For this review, take the finished solid that the model builds, in its own axes (mm). A direction names the side the tool comes from. Round coordinates to 2 decimals unless told otherwise and drop trailing zeros. Write each loop counter-clockwise with the first axis right and the second up, starting at its lowest first coordinate (ties: lowest second). Pieces come first, ordered by that corner, then holes.
from build123d import *

# Parameters (mm, degrees)
F0_W     = 42.5292160362
F0_H     = 54.7678396106
F1_DEPTH = 25.4
F5_DEPTH = 12.7
F6_DEPTH = 12.7


with BuildPart() as f1:
    # F0 (on Right) → F1 (new body)
    with BuildSketch(Plane.YZ):
        with Locations((0.3059664741, 8.7200179696)):
            Rectangle(F0_W, F0_H)
    extrude(amount=F1_DEPTH)


with BuildPart() as f5:
    # F4 (on Front) → F5 (new body, symmetric)
    with BuildSketch(Plane.XZ):
        Polygon((7.8021222726, 46.5067662299), (-7.8021222726, 46.5067662299), (-15.1452962309, 44.0590418875), (-23.1004003435, 35.4920066893), (-25.8540920913, 30.2905943245), (-27.6898853481, 19.5817966014), (-27.3839198053, 5.8133457787), (-30.1376096904, 8.8730016723), (-32.5853340328, 7.9551050439), (-34.4211272895, 4.5894836076), (-34.1151617467, -1.8357934896), (-33.1972651184, -7.3431739584), (-30.4435752332, -11.6266915575), (-27.0779542625, -12.85055466), (-26.1600576341, -18.6639018357), (-23.7123332918, -24.7832108289), (-17.2870550305, -33.3502478898), (-10.8617777005, -43.1411489844), (-5.9663290158, -45.8948388696), (0.1529839792, -47.1187010407), (5.6603644043, -45.5888696015), (11.4582879852, -42.2321807174), (17.2870550305, -33.3502478898), (22.4884822373, -26.4150121165), (24.2018731435, -23.5593615721), (26.1600576341, -18.6639018357), (26.5130960305, -16.4279912753), (26.4660250396, -15.9102100879), (26.6190057487, -15.7572295118), (27.0779542625, -12.85055466), (30.4435752332, -11.6266915575), (33.1972651184, -7.3431739584), (34.1151617467, -1.8357934896), (34.4211272895, 4.5894836076), (32.5853340328, 7.9551050439), (31.7694234351, 8.2610715181), (29.5868726354, 8.2610715181), (27.3839198053, 5.8133457787), (27.6898853481, 19.5817966014), (25.8540920913, 30.2905943245), (23.1004003435, 35.4920066893), (15.1452962309, 44.0590418875), align=None)
    extrude(amount=F5_DEPTH, both=True)

    # F3 (on Right) → F6 (join, symmetric)
    with BuildSketch(Plane.YZ):
        Polygon((-16.6751239449, 46.2008044124), (-39.0106141567, 19.8877640069), (-39.6225452423, 19.8877640069), (-37.1748209, 14.6863479167), (-34.1151617467, 5.8133457787), (-28.3018164337, -3.6715869792), (-22.4884711206, -15.6042445451), (-11.1677432433, -24.4772471488), (-1.3768438948, -33.0442860723), (10.555813089, -40.6934246421), (23.4063696116, -45.282907784), (28.6077857018, -46.2008044124), (31.9734066725, -46.2008044124), (34.115165472, -43.4471108019), (38.7046486139, -31.2084890902), (39.0106141567, -28.7607647479), (37.1748209, -28.4547992051), (37.7867519855, -26.9249714911), (36.2569242716, -17.7460033447), (39.6225452423, -17.4400378019), (43.2941317558, -15.6042445451), (42.6822006702, -13.1565211341), (39.6225452423, -10.4028293863), (40.2344763279, -10.7087958604), (34.4211310148, 1.2238622876), (35.9509587288, 7.3431739584), (31.6674411297, 18.0519688874), (29.9477812825, 26.3130422682), (29.9477812825, 31.1950890951), (31.6674411297, 34.8800756037), (13.3095029742, 43.4471108019), (4.7424673103, 43.4471108019), align=None)
    extrude(amount=F6_DEPTH, both=True)


solid = f5.part
(1) For line 1 along X through (y, z) = (24, 2.5); line 2 along Y through (x, z) = (4, -27), list the stretches that pass through material, from the lowest coordinate up.
Geometry check:
line 1: x = -12.7 to 12.7
line 2: y = -12.7 to 37.76
(2) For pin 1 Ø2.5 at (x, z) = (-1, 29) entering from +Y; pin 2 Ø0.7 at (x, z) = (0.5, 46) entering from -Y; pin 3 Ø10 at (x, z) = (0, 0) entering from -Y, all flat-tipped, find the tip position at first contact; note any pin that passes through.
Geometry check:
pin 1: stops at y = 29.95
pin 2: stops at y = -17.14
pin 3: stops at y = -33.62
(3) We need section B-B, the plane x = -19.5. Give the boundary of the cut face in (y, z).
Geometry check:
outline: (-12.7, -30.4) - (12.7, -30.4) - (12.7, 39.37) - (-12.7, 39.37) - close
(4) We need section C-C, the plane y = -20. Give the boundary of the cut face in (x, z), and give its area (3 significant figures).
Geometry check:
outline: (-12.7, -17.55) - (12.7, -17.55) - (12.7, 42.28) - (-12.7, 42.28) - close
area: 1,520 mm2
(5) We need section A-A, the plane z = 37.5. Give the boundary of the cut face in (x, y), and give its area (3 significant figures).
Geometry check:
outline: (-21.24, -12.7) - (-12.7, -12.7) - (-12.7, -24.06) - (12.7, -24.06) - (12.7, -12.7) - (21.24, -12.7) - (21.24, 12.7) - (12.7, 12.7) - (12.7, 26.05) - (-12.7, 26.05) - (-12.7, 12.7) - (-21.24, 12.7) - close
area: 1,710 mm2
(6) Mouldability with a two-part tool opening along Z and no side actions: class faces 1 (the face through (26.785, -0.178, 24.861)), 2 (the face through (0.178, 37.033, -22.4)), 3 (the face through (0.18, -17.66, -19.39)) as pulls with the +Z half, pulls with the -Z half, needs draft (parallel to the pull), parting line crosses it, or undercut.
Geometry check:
face 1: pulls with the +Z half
face 2: undercut
face 3: pulls with the -Z half
(7) For faces 4 (the face through (-14.119, -0.178, -38.177)), 5 (the face through (-34.27, -0.18, 1.42)), list the 3-axis set-ups (+Z, -Z, +X, -X, +Y, -Y) from which the entire face can be reached by the end or side of a thin tool; tool diameter is ignored.
Geometry check:
face 4: -Z, -X, -Y
face 5: -Z, -X, +Y, -Y
